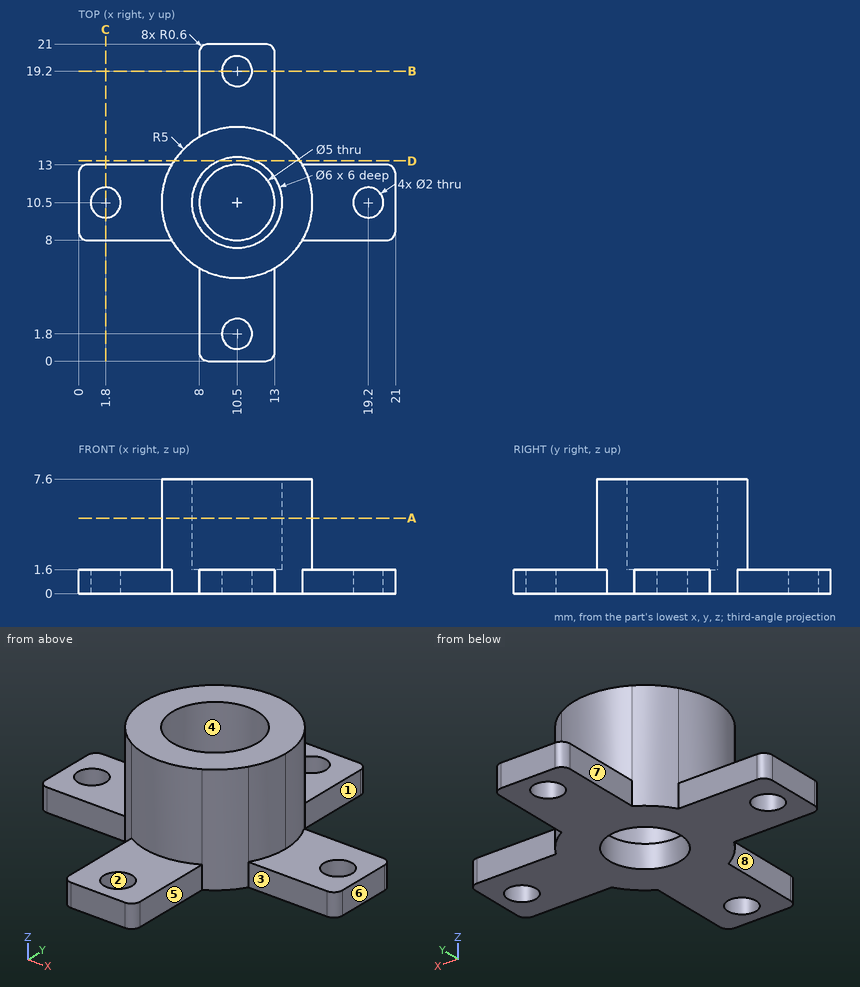
Geometry: see drawing. Coordinates: mm, zero at the bounding-box minimum. A direction names the side the tool comes from. Round coordinates to 2 decimals unless told otherwise and drop trailing zeros. Loops run counter-clockwise (first coordinate to the right, second up) from the corner with the lowest first, then second, coordinate; pieces in that order, holes last.
(1) Contact query for flat-ended pins moving along their axis: pin 1 Ø4 at (x, z) = (16, 2.5) entering from -Y; pin 2 Ø2.5 at (x, y) = (2.5, 11) entering from +Z; pin 3 Ø3 at (y, z) = (15, 5) entering from -X. Output: stop coordinate, or through.
From the geometry:
pin 1: stops at y = 6.93
pin 2: stops at z = 1.6
pin 3: stops at x = 6.5
(2) Pull-direction query (Y, two-part tool) for the marked faces 1, 2 and 3; classes: +Y half, -Y half, draft (parallel to the pull), parting line (faces both ways), or undercut.
From the geometry:
face 1: draft
face 2: undercut
face 3: -Y half
(3) Section query A-A (z = 5). Output: boundary loops of the cut face in (x, y), and give its area (3 significant figures).
From the geometry:
outline: circle Ø10 at (10.5, 10.5); hole circle Ø6 at (10.5, 10.5)
area: 50.3 mm2
(4) Section query D-D (y = 13.25). Output: boundary loops of the cut face in (x, z), and give its area (3 significant figures).
From the geometry:
outline: (6.32, 0) - (14.68, 0) - (14.68, 7.6) - (11.7, 7.6) - (11.7, 1.6) - (9.3, 1.6) - (9.3, 7.6) - (6.32, 7.6) - close
area: 49.1 mm2
(5) Section query B-B (y = 19.2). Output: boundary loops of the cut face in (x, z).
From the geometry:
outline: (8, 0) - (9.5, 0) - (9.5, 1.6) - (8, 1.6) - close; (11.5, 0) - (13, 0) - (13, 1.6) - (11.5, 1.6) - close
(6) Material intervals for probe 1 along Y at (x, z) = (10.5, 0.55); probe 2 along Z at (x, y) = (11, 17.5); probe 3 along Y at (x, z) = (19.2, 0.45), sorted ascending.
From the geometry:
probe 1: y = 0 to 0.8, 2.8 to 8, 13 to 18.2, 20.2 to 21
probe 2: z = 0 to 1.6
probe 3: y = 8 to 9.5, 11.5 to 13
(7) Access query for the marked faces 4, 5, 6, 7 and 8. Directions: +Z, -Z, +X, -X, +Y, -Y. A direction counts if a zero-diameter tool reaches every point of the face in a straight line with its end or side. Return the directions, or none.
From the geometry:
face 4: +Z
face 5: +Z, -Z, +X, -Y
face 6: +Z, -Z, +X, +Y, -Y
face 7: +Z, -Z, -X, +Y
face 8: +Z, -Z, -X, -Y
